Geometry check sheet. Reference: the model listing, model coordinates, mm. Face numbers are marked on the shaded views. Give positions to 0.01 mm unless a question says otherwise; leave off trailing zeros. Loops run counter-clockwise (first coordinate to the right, second up) from the corner with the lowest first, then second, coordinate; pieces in that order, holes last. Notation, with made-up numbers: (77, -15) - (114, -15) arc R24 cw to (114, 4) - close; hole circle Ø6 at (-10, 16). An arc over 180 degrees is marked (long way). Write item = value, one per line. Start each with the question number.
from build123d import *

# Parameters (mm, degrees)
SKETCH003_W     = 35.78
SKETCH003_H     = 41.185
PAD002_DEPTH    = 4
SKETCH004_W     = 19.78
SKETCH004_H     = 39.185
POCKET003_DEPTH = 2
SKETCH006_R     = 1.1
POCKET005_DEPTH = 4.001
SKETCH007_R     = 2.25
POCKET006_DEPTH = 2
CHAMFER001_SIZE = 1
SKETCH019_W     = 19.78
SKETCH019_H     = 2
POCKET015_DEPTH = 2


with BuildPart() as part:
    # Sketch003 (on ShapeBinder) → Pad002 (new body)
    with BuildSketch(Plane(origin=(0, 0, 0), x_dir=(1, 0, 0), z_dir=(0, 0, -1))):
        with Locations((76.18, 45.1675)):
            Rectangle(SKETCH003_W, SKETCH003_H)
    extrude(amount=PAD002_DEPTH)

    # Sketch004 (on ShapeBinder) → Pocket003 (cut)
    with BuildSketch(Plane(origin=(0, 0, 0), x_dir=(1, 0, 0), z_dir=(0, 0, -1))):
        with Locations((76.18, 44.1675)):
            Rectangle(SKETCH004_W, SKETCH004_H)
    extrude(amount=POCKET003_DEPTH, mode=Mode.SUBTRACT)

    # Sketch006 (on Face4 of Pocket003) → Pocket005 (cut, through all)
    with BuildSketch(Plane.XY):
        with Locations((62.29, -32.575)):
            Circle(SKETCH006_R)
        with Locations((90.07, -32.575)):
            Circle(SKETCH006_R)
        with Locations((90.07, -55.76)):
            Circle(SKETCH006_R)
        with Locations((62.29, -55.76)):
            Circle(SKETCH006_R)
    extrude(amount=-POCKET005_DEPTH, mode=Mode.SUBTRACT)

    # Sketch007 (on Face5 of Pocket005) → Pocket006 (cut)
    with BuildSketch(Plane(origin=(0, 0, -4), x_dir=(1, 0, 0), z_dir=(0, 0, -1))):
        with Locations((62.29, 55.76)):
            Circle(SKETCH007_R)
        with Locations((90.07, 55.76)):
            Circle(SKETCH007_R)
        with Locations((90.07, 32.575)):
            Circle(SKETCH007_R)
        with Locations((62.29, 32.575)):
            Circle(SKETCH007_R)
    extrude(amount=-POCKET006_DEPTH, mode=Mode.SUBTRACT)

    # Chamfer001
    chamfer001_edges = [part.edges().sort_by_distance(p)[0] for p in [
        (76.18, -65.76, -4),
        (94.07, -45.1675, -4),
        (58.29, -45.1675, -4),
        (58.29, -65.76, -2),
        (94.07, -65.76, -2),
    ]]
    chamfer(chamfer001_edges, length=CHAMFER001_SIZE)

    # Sketch019 (on Face7 of Chamfer001) → Pocket015 (cut)
    with BuildSketch(Plane(origin=(0, -24.575, 0), x_dir=(-1, 0, 0), z_dir=(0, 1, 0))):
        with Locations((-76.18, -3)):
            Rectangle(SKETCH019_W, SKETCH019_H)
    extrude(amount=-POCKET015_DEPTH, mode=Mode.SUBTRACT)


solid = part.part
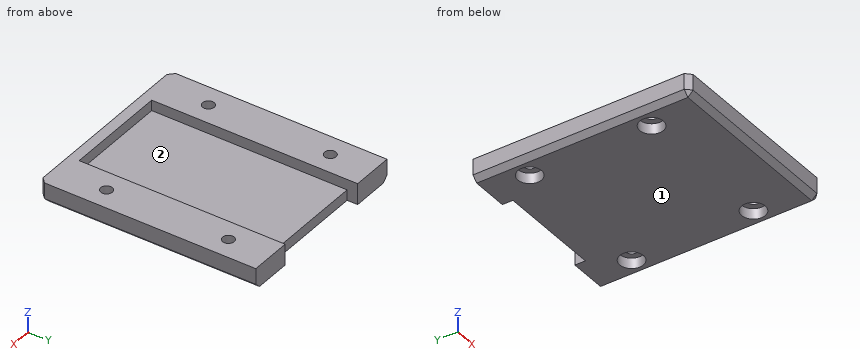
1) Cross-section at A-A on y = -55.76. Enter the section's corners in (x, z), and give its area (3 significant figures).
2) Gauge pin test, flat ends, axial feed: P1, Ø8, axis at x = 75.5, y = -56, coming from the +Z side; P2, Ø1.8, axis at x = 90.07, y = -32.575, coming from the +Z side; P3, Ø2, axis at x = 63, y = -55, coming from the -Z side. Record the tip position at first contact, or that the pin passes through.
3) Cross-section at D-D on x = 78. Enter the section's corners in (y, z) (3 decimals).
4) Release check for a two-part mould opening along X. For the marked faces 1 and 2 record: pulls with the +X half, pulls with the -X half, needs draft (parallel to the pull), parting line crosses it, or undercut.
5) Cross-section at B-B on x = 90.07. Enter the section's corners in (y, z) (3 decimals), and give its area (3 significant figures).
6) Material ranges on line 1 along X through (y, z) = (-55.76, -2.5); line 2 along Y through (x, z) = (62.29, -2.65) (3 decimals); line 3 along Y through (x, z) = (62.29, -1) (3 decimals), recorded low to high.
7) Cross-section at C-C on y = -43. Enter the section's corners in (x, z), and give its area (3 significant figures).
Checked values:
q1.outline = (58.29, -3) - (59.29, -4) - (60.04, -4) - (60.04, -2) - (61.19, -2) - (61.19, 0) - (58.29, 0) - close; (63.39, -2) - (64.54, -2) - (64.54, -4) - (87.82, -4) - (87.82, -2) - (88.97, -2) - (88.97, 0) - (86.07, 0) - (86.07, -2) - (66.29, -2) - (66.29, 0) - (63.39, 0) - close; (91.17, -2) - (92.32, -2) - (92.32, -4) - (93.07, -4) - (94.07, -3) - (94.07, 0) - (91.17, 0) - close
q1.area = 75.8 mm²
q2.P1 = -2
q2.P2 = through
q2.P3 = -2
q3.outline = (-65.76, -3) - (-64.76, -4) - (-26.575, -4) - (-26.575, -2) - (-63.76, -2) - (-63.76, 0) - (-65.76, 0) - close
q4.face_1 = needs draft
q4.face_2 = undercut
q5.outline = (-65.76, -3) - (-64.76, -4) - (-58.01, -4) - (-58.01, -2) - (-56.86, -2) - (-56.86, 0) - (-65.76, 0) - close; (-54.66, -2) - (-53.51, -2) - (-53.51, -4) - (-34.825, -4) - (-34.825, -2) - (-33.675, -2) - (-33.675, 0) - (-54.66, 0) - close; (-31.475, -2) - (-30.325, -2) - (-30.325, -4) - (-24.575, -4) - (-24.575, 0) - (-31.475, 0) - close
q5.area = 137 mm²
q6.line_1 = 58.29 to 60.04, 64.54 to 87.82, 92.32 to 94.07
q6.line_2 = -65.76 to -58.01, -53.51 to -34.825, -30.325 to -24.575
q6.line_3 = -65.76 to -56.86, -54.66 to -33.675, -31.475 to -24.575
q7.outline = (58.29, -3) - (59.29, -4) - (93.07, -4) - (94.07, -3) - (94.07, 0) - (86.07, 0) - (86.07, -2) - (66.29, -2) - (66.29, 0) - (58.29, 0) - close
q7.area = 103 mm²
